Design review of the part built by this model. Coordinates are the model's own, in mm. A direction names the side the tool comes from. Round coordinates to 2 decimals unless told otherwise and drop trailing zeros. Loops run counter-clockwise (first coordinate to the right, second up) from the corner with the lowest first, then second, coordinate; pieces in that order, holes last. Notation, with made-up numbers: (0.5, 10) -> (47.5, 10) arc R25 cw to (47.5, 42) -> close; hole circle Ø11 at (61.5, 87.5). An arc over 180 degrees is marked (long way). Answer as CSV lines item,"result". Start each with the question number.
(1) Take a section at D-D, the plane y = 2.5. State how many separate pieces and enclosed holes the cut face has, and give its area (4 significant figures).
(2) Draft analysis for pull direction X (two halves, no side actions). For faces 1 (the face through (4, -4, -2.5)), 2 (the face through (-13.887, -10.648, 0.035)), 3 (the face through (-0.202, -0.048, -25.037)), state which applies: +X half, -X half, draft (parallel to the pull), parting line (faces both ways), or undercut.
(3) Take a section at A-A, the plane z = -15.5. Write out the cut boundary in (x, y), and give its area (3 significant figures).
(4) Take a section at B-B, the plane z = 14. Write out the cut boundary in (x, y).
(5) Machinability: for faces 4 (the face through (-0.867, 3.905, -6.049)), 5 (the face through (-0.12, 15.75, 6.44)), 6 (the face through (-1.49, 2.64, 23.95)), 7 (the face through (3.014, -1.708, -19.36)), which of the approach directions +Z, -Z, +X, -X, +Y, -Y give a long, thin tool a straight path to every point of the face, cutting with its end or side? Answer none if there is none.
(6) For P1, Ø2.5, axis at x = 0, z = -15.5, coming from the +Y side; P2, Ø12, axis at y = -5, z = 12, coming from the +X side; P3, Ø4, axis at x = 3, y = 10.5, coming from the +Z side; P4, Ø8, axis at x = 7.5, y = 8.5, coming from the -Z side, all flat-tipped, find the tip position at first contact; note any pin that passes through.
(7) Take a section at C-C, the plane x = 14.5. Write out the cut boundary in (y, z), and give its area (3 significant figures).
(8) To check wall thickness, follow line 1 (Z direction, x = 0, y = 0); line 2 (Z direction, x = 0, y = -1.25); line 3 (X direction, y = 0.5, z = -15.5). State the ranges of each line that lie inside material, in increasing order. Write a range as from..to.
from build123d import *

# Parameters (mm, degrees)
SKETCH1_R           = 17.5
BOSS_EXTRUDE1_DEPTH = 2.5
BOSS_EXTRUDE2_DEPTH = 8
SKETCH3_R           = 4
BOSS_EXTRUDE3_DEPTH = 18
BOSS_EXTRUDE4_START = 7
SKETCH7_R           = 4
BOSS_EXTRUDE4_DEPTH = 7
BOSS_EXTRUDE5_DEPTH = 20
SKETCH10_R          = 1.55
CUT_EXTRUDE1_DEPTH  = 7
BOSS_EXTRUDE6_DEPTH = 7
SKETCH12_R          = 1.55
CUT_EXTRUDE2_DEPTH  = 6.1


with BuildPart() as part:
    # Sketch1 → Boss-Extrude1 (new, symmetric)
    with BuildSketch(Plane.XY):
        Circle(SKETCH1_R)
    extrude(amount=BOSS_EXTRUDE1_DEPTH, both=True)

    # Sketch2 → Boss-Extrude2 (add)
    with BuildSketch(Plane.XY.offset(2.5)):
        with BuildLine():
            Line((7.875, 13.63990011), (4.125, 7.144709581))
            ThreePointArc((4.125, 7.144709581), (0, 8.25), (-4.125, 7.144709581))
            Line((-4.125, 7.144709581), (-7.875, 13.63990011))
            ThreePointArc((-7.875, 13.63990011), (0, 15.75), (7.875, 13.63990011))
        make_face()
    extrude(amount=BOSS_EXTRUDE2_DEPTH)

    # Sketch3 → Boss-Extrude3 (add)
    with BuildSketch(Plane.XY.offset(2.5)):
        Circle(SKETCH3_R)
    extrude(amount=BOSS_EXTRUDE3_DEPTH)

    # Sketch7 → Boss-Extrude4 (add)
    with BuildSketch(Plane(origin=(0, 0, -2.5), x_dir=(-1, 0, 0), z_dir=(0, 0, -1)).offset(BOSS_EXTRUDE4_START)):
        with Locations(Location((0, 0, 0), (0, 0, 180))):
            Circle(SKETCH7_R)
    extrude(amount=-BOSS_EXTRUDE4_DEPTH)

    # Sketch9 → Boss-Extrude5 (add)
    with BuildSketch(Plane(origin=(0, 0, -9.5), x_dir=(-1, 0, 0), z_dir=(0, 0, -1))):
        Polygon((4, 0), (2, 3.464101615), (-2, 3.464101615), (-4, 0), (-2, -3.464101615), (2, -3.464101615), align=None)
    extrude(amount=BOSS_EXTRUDE5_DEPTH)

    # Sketch10 → Cut-Extrude1 (cut)
    with BuildSketch(Plane(origin=(0, -3.464101615, 0), x_dir=(-1, 0, 0), z_dir=(0, 1, 0))):
        with Locations(Location((0, -23.5, 0), (0, 0, 180))):
            Circle(SKETCH10_R)
        with Locations(Location((0, -15.5, 0), (0, 0, 180))):
            Circle(SKETCH10_R)
    extrude(amount=CUT_EXTRUDE1_DEPTH, mode=Mode.SUBTRACT)

    # Sketch11 → Boss-Extrude6 (add)
    with BuildSketch(Plane.XY.offset(20.5)):
        Polygon((3.031088913, 1.75), (0, 3.5), (-3.031088913, 1.75), (-3.031088913, -1.75), (0, -3.5), (3.031088913, -1.75), align=None)
    extrude(amount=BOSS_EXTRUDE6_DEPTH)

    # Sketch12 → Cut-Extrude2 (cut)
    with BuildSketch(Plane(origin=(-1.515544457, -2.625, 0), x_dir=(0.8660254037844372, -0.5000000000000026, 0), z_dir=(-0.5000000000000026, -0.8660254037844372, 0))):
        with Locations((0, 24)):
            Circle(SKETCH12_R)
    extrude(amount=-CUT_EXTRUDE2_DEPTH, mode=Mode.SUBTRACT)


solid = part.part
The answers:
1,separate pieces,"1"
1,enclosed holes,"2"
1,area,"435.5 mm²"
2,face 1,"draft"
2,face 2,"parting line"
2,face 3,"undercut"
3,outline,"(-4, 0) -> (-2, -3.46) -> (-1.55, -3.46) -> (-1.55, 3.46) -> (-2, 3.46) -> close; (1.55, -3.46) -> (2, -3.46) -> (4, 0) -> (2, 3.46) -> (1.55, 3.46) -> close"
3,area,"20.1 mm²"
4,outline,"circle Ø8 at (0, 0)"
5,face 4,"-Z"
5,face 5,"+Z, +Y"
5,face 6,"+Z, -X, +Y"
5,face 7,"-Z, +X, -Y"
6,P1,"through"
6,P2,"x = 4"
6,P3,"z = 10.5"
6,P4,"z = -2.5"
7,outline,"(-9.8, -2.5) -> (9.8, -2.5) -> (9.8, 2.5) -> (-9.8, 2.5) -> close"
7,area,"98.0 mm²"
8,line 1,"-29.5..-25.05, -21.95..-17.05, -13.95..22.45, 25.55..27.5"
8,line 2,"-29.5..-25.05, -21.95..-17.05, -13.95..22.58, 25.42..27.5"
8,line 3,"-3.71..-1.55, 1.55..3.71"
